For this review, take the finished solid that the model builds, in its own axes (mm). A direction names the side the tool comes from. Coordinates: 2 decimals unless noted, no trailing zeros. Write each loop counter-clockwise with the first axis right and the second up, starting at its lowest first coordinate (ties: lowest second). Pieces come first, ordered by that corner, then holes. Notation, with made-up numbers: (35, 40) -> (49, 40) arc R21 ccw to (49, 67) -> close; hole circle Ø8 at (65, -24). An arc over 180 degrees is marked (long way). Put each result on its own line as item: value. Start each with the question number.
Item 1: The part is to be moulded in two halves that separate along X. For faces 4 (the flat face through (0, 1.27, 0)), 5 (the flat face through (1, 0, 0)), 6 (the conical face through (1.77, 0.18, 0.03)), say which applies: +X half, -X half, draft (parallel to the pull), parting line (faces both ways), or undercut.
Item 2: To check wall thickness, follow L1, parallel to Y at x = -1.65, z = 1.45; L2, parallel to X at y = 10, z = -0.7; L3, parallel to Z at x = 1.85, y = 2. State the ranges of each line that lie inside material, in increasing order.
Item 3: Insertion check: P1, Ø1, axis at y = 3.5, z = -1, coming from the -X side; P2, Ø1, axis at y = 0.5, z = 0, coming from the +X side; P3, Ø0.6, axis at x = 0, z = 0, coming from the -Y side. Each pin has a flat end and moves straight along its axis. Give the tip position at first contact, or say it passes through.
Item 4: Consider section D-D on y = 5.5. Give the boundary of the cut face in (x, z), and give its area (3 significant figures).
Item 5: Consider section C-C on y = 13.5. Give the boundary of the cut face in (x, z), and give its area (3 significant figures).
Item 6: For faces 1 (the flat face through (0.635, 1, 0)), 2 (the cylindrical face through (-1.94, 6.52, -0.61)), 3 (the conical face through (-1.77, 0.18, -0.03)), list the 3-axis set-ups (+Z, -Z, +X, -X, +Y, -Y) from which the entire face can be reached by the end or side of a thin tool; tool diameter is ignored.
Autodesk Inventor part; units mm, degrees
ref_plane "YZ Plane" through (0, 0, 0) normal (1, 0, 0) x (0, 1, 0)
ref_plane "XZ Plane" through (0, 0, 0) normal (0, 1, 0) x (-1, 0, 0)
ref_plane "XY Plane" through (0, 0, 0) normal (0, 0, 1) x (1, 0, 0)
sketch "Sketch1" plane through (0, 0, 0) normal (0, 1, 0) x (-1, 0, 0)
  circle A0 centre (0, 0) radius 2.032
  line L0 (-0.635, 2.032) -> (0.635, 2.032)
  line L1 (0.635, 2.032) -> (0.635, -2.032)
  line L2 (0.635, -2.032) -> (-0.635, -2.032)
  line L3 (-0.635, -2.032) -> (-0.635, 2.032)
  line L4 (-0.635, 2.032) -> (0.635, -2.032) construction
  line L5 (0.635, 2.032) -> (-0.635, -2.032) construction
  dimension "d0" = 4.064
  dimension "d10" = 1.27
extrude "Extrusion1" add sketch "Sketch1" along normal blind 12.954 contours A0 L1 | L1 A0 L3 | L3 A0
sketch "Sketch2" plane through (0, 12.954, 0) normal (0, 1, 0) x (1, 0, 0)
  circle A0 centre (0, 0) radius 2.413
  dimension "d5" = 4.826
extrude "Extrusion2" add sketch "Sketch2" along normal blind 6.1595
thread "Thread2"
chamfer "Chamfer1" distance 0.381 angle 45 1 edges at (2.032, 12.954, 0)
chamfer "Chamfer2" distance 1.27 angle 20 1 edges at (-2.413, 19.1135, 0) measured on face at (2.4052, 17.0603, 0.1942)
chamfer "Chamfer3" distance 0.635 angle 30 1 edges at (2.032, 0, 0) measured on face at (-2.0254, 8.3823, -0.1635)
extrude "Extrusion3" cut sketch "Sketch1" along normal blind 1.27 contours L1 A0 L3 | A0 L0 L1 | L1 L2 A0 | A0 L3 L0 | L2 L3 A0
properties part number "0.16 Shaft" material "Stainless Steel"
Return value:
1. face 4: undercut
1. face 5: draft
1. face 6: +X half
2. L1: 12.74 to 18.44
2. L2: -1.91 to 1.91
2. L3: -0.84 to 0.84
3. P1: x = -1.97
3. P2: x = 2.03
3. P3: y = 1.27
4. outline: circle Ø4.06 at (0, 0)
4. area: 13.0 mm^2
5. outline: circle Ø4.83 at (0, 0)
5. area: 18.3 mm^2
6. face 1: +Z, -Z, -Y
6. face 2: -Y
6. face 3: -X, -Y
